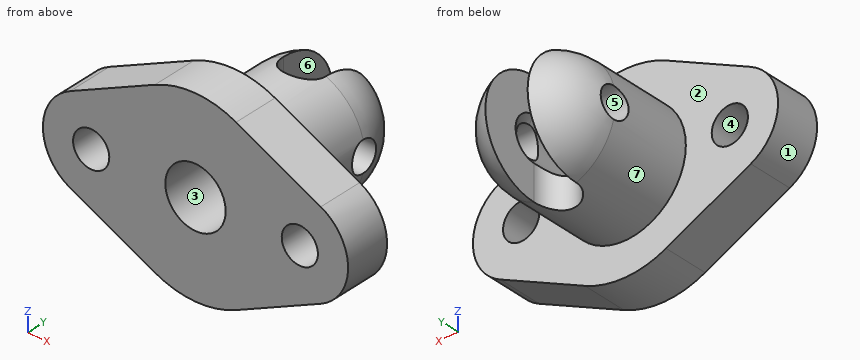
from build123d import *

# Parameters (mm, degrees)
SKETCH1_R               = 6.000000000045659
SKETCH1_R_2             = 6.000000000000002
BOSS_EXTRUDE3_DEPTH     = 15
CUT_EXTRUDE1_DEPTH      = 86.80768734285536
CUT_EXTRUDE1_DEPTH_BACK = 86.80768734285536
CUT_EXTRUDE2_DEPTH      = 85.89816666292398
CUT_EXTRUDE2_DEPTH_BACK = 85.89816666292398
SKETCH8_R               = 4.999999999999999


with BuildPart() as part:
    # Sketch1 → Boss-Extrude3 (new body)
    with BuildSketch(Plane(origin=(0, 0, 0), x_dir=(1, 0, 0), z_dir=(0, 1, 0))):
        with BuildLine():
            Line((13.448529411746133, -27.930933687605208), (41.51744765706708, -14.415965774247848))
            ThreePointArc((41.51744765706708, -14.415965774247848), (50.57627118648844, 3.55e-15), (41.51744765706708, 14.415965774247855))
            Line((41.51744765706708, 14.415965774247855), (13.448529411746131, 27.930933687605208))
            ThreePointArc((13.448529411746131, 27.930933687605208), (1.9e-15, 31.000000000000004), (-13.448529411746135, 27.930933687605208))
            Line((-13.448529411746135, 27.930933687605208), (-41.51744765706708, 14.415965774247852))
            ThreePointArc((-41.51744765706708, 14.415965774247852), (-50.576271186488434, 1.96e-15), (-41.51744765706708, -14.415965774247852))
            Line((-41.51744765706708, -14.415965774247852), (-13.448529411746136, -27.93093368760521))
            ThreePointArc((-13.448529411746136, -27.93093368760521), (1.9e-15, -31.000000000000007), (13.448529411746133, -27.930933687605208))
        make_face()
        with Locations(Location((-34.57627118648843, 0, 0), (0, 0, 270))):
            Circle(SKETCH1_R, mode=Mode.SUBTRACT)
        with Locations(Location((34.57627118648844, 0, 0), (0, 0, 270))):
            Circle(SKETCH1_R_2, mode=Mode.SUBTRACT)
    extrude(amount=BOSS_EXTRUDE3_DEPTH)

    # Sketch5 → Revolve1 (revolve)
    with BuildSketch(Plane.XY):
        with BuildLine():
            Line((0, 0), (0, 42))
            Line((0, 42), (-6.983e-14, 62.00000000000001))
            ThreePointArc((-6.983e-14, 62.00000000000001), (-14.14213562373098, 56.14213562373093), (-20, 42))
            Line((-20, 42), (-19.999999999999996, 0))
            Line((-19.999999999999996, 0), (0, 0))
        make_face()
    revolve(axis=Axis((0, 0, 0), (0, 1, 0)))

    # Sketch6 → Cut-Revolve1 (revolve, cut)
    with BuildSketch(Plane.XY):
        with BuildLine():
            Line((-1.73e-15, 0), (0, 42))
            Line((0, 42), (0, 52.00000000000001))
            ThreePointArc((0, 52.00000000000001), (-7.07106781186548, 49.07106781186548), (-9.999999999999998, 42))
            Line((-9.999999999999998, 42), (-9.999999999999995, 2.1e-16))
            Line((-9.999999999999995, 2.1e-16), (-1.73e-15, 0))
        make_face()
    revolve(axis=Axis((-1.73e-15, 0, 0), (4e-17, 1, 0)), mode=Mode.SUBTRACT)

    # Sketch7 → Cut-Extrude1 (cut, two sides: drawn at the far end of the back side and taken through both)
    with BuildSketch(Plane.XY.offset(-CUT_EXTRUDE1_DEPTH_BACK)):
        with BuildLine():
            Line((-6.999999999999999, 42), (-6.999999999999999, 60.734993995195204))
            ThreePointArc((-6.999999999999999, 60.734993995195204), (1.22e-15, 62.00000000000001), (6.999999999999999, 60.734993995195204))
            Line((6.999999999999999, 60.734993995195204), (6.999999999999999, 42))
            ThreePointArc((6.999999999999999, 42), (-1.29e-15, 35), (-6.999999999999999, 42))
        make_face()
    extrude(amount=CUT_EXTRUDE1_DEPTH + CUT_EXTRUDE1_DEPTH_BACK, mode=Mode.SUBTRACT)

    # Sketch8 → Cut-Extrude2 (cut, two sides: drawn at the far end of the back side and taken through both)
    with BuildSketch(Plane(origin=(0, 0, 0), x_dir=(0, 0, -1), z_dir=(1, 0, 0)).offset(-CUT_EXTRUDE2_DEPTH_BACK)):
        with Locations((3.47e-15, 42)):
            Circle(SKETCH8_R)
    extrude(amount=CUT_EXTRUDE2_DEPTH + CUT_EXTRUDE2_DEPTH_BACK, mode=Mode.SUBTRACT)


solid = part.part
CAD build for the part. Positions are in the model's coordinates, mm. Face numbers are marked on the shaded views. A direction names the side the tool comes from. Round coordinates to 2 decimals unless told otherwise and drop trailing zeros. Loops run counter-clockwise (first coordinate to the right, second up) from the corner with the lowest first, then second, coordinate; pieces in that order, holes last. Notation, with made-up numbers: M 23.25,5 L 31.25,5 A12 cw 31.25,23 Z; hole C 73,48 d9. An arc over 180 degrees is marked long. One line per question, with ' | ' between items. Start each with the question number.
Item 1: Wall check: line 1 (X direction, y = 3, z = 0); line 2 (X direction, y = 33, z = 0); line 3 (Y direction, x = -37.5, z = -10.5). Give the ranges that are in metal, low to high.
Item 2: Cut at A-A, the plane x = 0. Write the cut outline in (y, z), plus the area to 3 significant figures.
Item 3: Cut at C-C, the plane y = 44. Write the cut outline in (x, z).
Item 4: Cut at D-D, the plane x = 15. Write the cut outline in (y, z), plus the area to 3 significant figures.
Item 5: Cut at B-B, the plane z = 0. Write the cut outline in (x, y) (3 decimals).
Item 6: Two-plate mould, pull along Z, no slides. Class the marked faces 1, 2, 3 and 4: pulls with the +Z half, pulls with the -Z half, needs draft (parallel to the pull), parting line crosses it, or undercut.
Item 7: Which spindle directions (+Z, -Z, +X, -X, +Y, -Y) get a long thin tool onto all of the face, cutting with end or side? Do the marked faces 5, 6 and 7. Say none if no direction does.
Item 8: Pin check, flat tips, straight feed: pin 1 Ø3 at (y, z) = (26.5, 10) entering from +X; pin 2 Ø10 at (y, z) = (44.5, -22) entering from -X; pin 3 Ø16 at (y, z) = (42, 0) entering from +X; pin 4 Ø12 at (x, z) = (0, 0) entering from -Y. Stop position of each tip, or through.
Responses:
1) line 1: x = -50.58 to -40.58, -28.58 to -10, 10 to 28.58, 40.58 to 50.58 | line 2: x = -20 to -10, 10 to 20 | line 3: y = 0 to 15
2) outline: M 0,-31 L 15,-31 L 15,-20 L 35,-20 L 35,-10 L 0,-10 Z; M 0,10 L 35,10 L 35,20 L 15,20 L 15,31 L 0,31 Z | area: 1,030 mm²
3) outline: M -19.36,-4.58 A19.9 ccw -7,-18.63 L -7,-6.86 A9.8 cw -8.66,-4.58 Z; M -19.36,4.58 L -8.66,4.58 A9.8 cw -7,6.86 L -7,18.63 A19.9 ccw Z; M 7,-18.63 A19.9 ccw 19.36,-4.58 L 8.66,-4.58 A9.8 cw 7,-6.86 Z; M 7,6.86 A9.8 cw 8.66,4.58 L 19.36,4.58 A19.9 ccw 7,18.63 Z
4) outline: M 0,-27.18 L 15,-27.18 L 15,-13.23 L 42,-13.23 A13.23 ccw 42,13.23 L 15,13.23 L 15,27.18 L 0,27.18 Z; hole C 42,0 d10 | area: 1,730 mm²
5) outline: M -50.576,0 L -40.576,0 L -40.576,15 L -50.576,15 Z; M -28.576,0 L -10,0 L -10,37 L -20,37 L -20,15 L -28.576,15 Z; M -19.365,47 L -8.66,47 A10 cw -7,49.141 L -7,60.735 A20 ccw Z; M 7,49.141 A10 cw 8.66,47 L 19.365,47 A20 ccw 7,60.735 Z; M 10,0 L 28.576,0 L 28.576,15 L 20,15 L 20,37 L 10,37 Z; M 40.576,0 L 50.576,0 L 50.576,15 L 40.576,15 Z
6) face 1: parting line crosses it | face 2: needs draft | face 3: undercut | face 4: undercut
7) face 5: +X, -X | face 6: +Z, -Z, +Y | face 7: +Y
8) pin 1: stops at x = 18.1 | pin 2: stops at x = -10.3 | pin 3: stops at x = 20 | pin 4: passes through
